Part model, mm, in its own coordinate system. Face numbers are marked on the shaded views. A direction names the side the tool comes from. Round coordinates to 2 decimals unless told otherwise and drop trailing zeros. Loops run counter-clockwise (first coordinate to the right, second up) from the corner with the lowest first, then second, coordinate; pieces in that order, holes last. Notation, with made-up numbers: M -21.5,-2.75 L -3.5,-2.75 A16 cw -3.5,16.25 Z; hole C 21,64 d10. An arc over 180 degrees is marked long. Put each result on its own line as item: value. Start each with the question number.
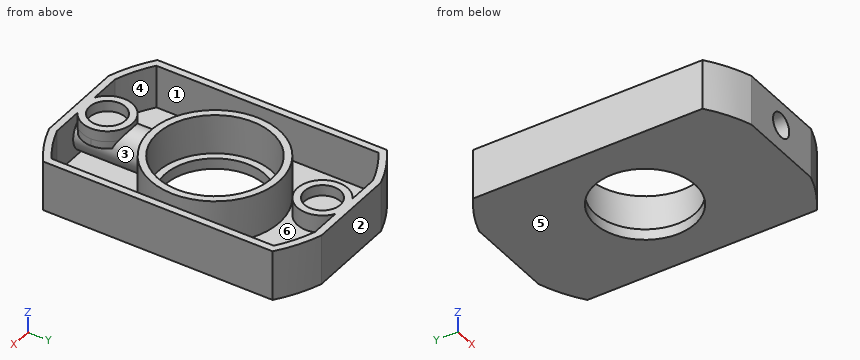
```python
from build123d import *

# Parameters (mm, degrees)
F0_R     = 20
F0_R_2   = 7
F1_DEPTH = 7
F2_R     = 8
F3_DEPTH = 5.5
F4_R     = 2.5
F5_DEPTH = 1.5
F7_DEPTH = 25
F8_R     = 1.7
F9_DEPTH = 10
F10_T    = 1


# Not quite as in the source:
# - a shell that OpenCascade refuses in one call is made with other operations: the cavity is built on its own and cut out


with BuildPart() as f1:
    # F0 (on Top) → F1 (new body)
    with BuildSketch(Plane.XY):
        Circle(F0_R)
        Circle(F0_R_2, mode=Mode.SUBTRACT)
    extrude(amount=F1_DEPTH)

    # F2 (on face) → F3 (cut)
    with BuildSketch(Plane.XY.offset(7)):
        Circle(F2_R)
    extrude(amount=-F3_DEPTH, mode=Mode.SUBTRACT)

    # F4 (on face) → F5 (cut)
    with BuildSketch(Plane.XY.offset(7)):
        with Locations((0, 15)):
            Circle(F4_R)
        with Locations((0, -15)):
            Circle(F4_R)
    extrude(amount=-F5_DEPTH, mode=Mode.SUBTRACT)

    # F6 (on face) → F7 (cut)
    with BuildSketch(Plane.XY.offset(7)):
        with BuildLine():
            Line((-12, -16), (-12, 16))
            ThreePointArc((-12, 16), (-20, 0), (-12, -16))
        make_face()
        with BuildLine():
            Line((12, 16), (12, 19))
            Line((12, 19), (6.2449979984, 19))
            ThreePointArc((6.2449979984, 19), (9.2449979984, 17.7349939952), (12, 16))
        make_face()
        with BuildLine():
            ThreePointArc((-12, 16), (-9.2449979984, 17.7349939952), (-6.2449979984, 19))
            Line((-6.2449979984, 19), (-12, 19))
            Line((-12, 19), (-12, 16))
        make_face()
        with BuildLine():
            Line((12, -19), (12, -16))
            ThreePointArc((12, -16), (9.2449979984, -17.7349939952), (6.2449979984, -19))
            Line((6.2449979984, -19), (12, -19))
        make_face()
        with BuildLine():
            ThreePointArc((-6.2449979984, -19), (-9.2449979984, -17.7349939952), (-12, -16))
            Line((-12, -16), (-12, -19))
            Line((-12, -19), (-6.2449979984, -19))
        make_face()
        with BuildLine():
            ThreePointArc((20, 0), (17.88854382, 8.94427191), (12, 16))
            Line((12, 16), (12, -16))
            ThreePointArc((12, -16), (17.88854382, -8.94427191), (20, 0))
        make_face()
        with BuildLine():
            Line((-6.2449979984, 19), (6.2449979984, 19))
            ThreePointArc((6.2449979984, 19), (0, 20), (-6.2449979984, 19))
        make_face()
        with BuildLine():
            ThreePointArc((-6.2449979984, -19), (0, -20), (6.2449979984, -19))
            Line((6.2449979984, -19), (-6.2449979984, -19))
        make_face()
    extrude(amount=-F7_DEPTH, mode=Mode.SUBTRACT)

    # F8 (on face) → F9 (cut)
    with BuildSketch(Plane.XZ.offset(19)):
        with Locations((0, 3.6865652073)):
            Circle(F8_R)
    extrude(amount=-F9_DEPTH, mode=Mode.SUBTRACT)

    # F10: shell of thickness 1, made by hand


with BuildPart() as f10_core1:
    # F10_t2: copy of F1
    add(f1.part)

    # the walls: a layer under each face that stays
    f10_faces = [f10_core1.faces().sort_by_distance(p)[0] for p in [
        (9.2449979984, 17.7349939952, 3.5),
        (-8, -12.6666666667, 0),
        (0, 19, 3.5),
        (12, 0, 3.5),
        (9.2449979984, -17.7349939952, 3.5),
        (4.1633319989, -19, 1.1666666667),
        (-9.2449979984, -17.7349939952, 3.5),
        (-12, 0, 3.5),
        (-9.2449979984, 17.7349939952, 3.5),
        (-7, 0, 0.75),
        (-2.5, -15, 6.25),
        (-8, 0, 4.25),
        (-2.5, 15, 6.25),
        (-1.7, -14, 3.6865652073),
        (-5.3333333333, -5.3333333333, 1.5),
        (0, -15, 5.5),
        (0, 15, 5.5),
        (0, -9, 3.6865652073),
    ]]
    thicken(f10_faces, amount=-F10_T, mode=Mode.SUBTRACT)

    # F10_s3 → F10_t4 (revolve, cut)
    with BuildSketch(Plane.XZ.offset(15)):
        Polygon((2.49, 5.51), (3.5, 5.5), (3.5, 4.5), (2.5, 4.5), align=None)
    revolve(axis=Axis((0, -15, 5.5), (0, 0, 1)), mode=Mode.SUBTRACT)

    # F10_s5 → F10_t6 (revolve, cut)
    with BuildSketch(Plane.XZ):
        Polygon((7.99, 1.51), (9, 1.5), (9, 0.5), (8, 0.5), align=None)
    revolve(axis=Axis((0, 0, 1.5), (0, 0, 1)), mode=Mode.SUBTRACT)

    # F10_s7 → F10_t8 (revolve, cut)
    with BuildSketch(Plane.XZ.offset(-15)):
        Polygon((2.49, 5.51), (3.5, 5.5), (3.5, 4.5), (2.5, 4.5), align=None)
    revolve(axis=Axis((0, 15, 5.5), (0, 0, 1)), mode=Mode.SUBTRACT)

    # F10_s9 → F10_t10 (revolve, cut)
    with BuildSketch(Plane.XY.offset(3.6865652073)):
        Polygon((1.69, -9.01), (2.7, -9), (2.7, -8), (1.7, -8), align=None)
    revolve(axis=Axis((0, -9, 3.6865652073), (0, -1, 0)), mode=Mode.SUBTRACT)


with BuildPart() as f1_1:
    add(f1.part)

    # what is left inside the walls is the cavity
    f10_cavity = [f10_core1.part.solids().sort_by_distance(p)[0] for p in [
        (5.5, -14, 1.01),
    ]]
    add(f10_cavity, mode=Mode.SUBTRACT)


solid = f1_1.part
```
1. Cut at C-C, the plane z = 3.25. Give the cut face in (x, y) (3 decimals), and give its area (3 significant figures).
2. Cut at B-B, the plane y = 0. Give the cut face in (x, z), and give its area (3 significant figures).
3. Cut at A-A, the plane y = 15. Give the cut face in (x, z), and give its area (3 significant figures).
4. Wall check: L1, parallel to Y at x = 0, z = 1.05; L2, parallel to Y at x = 0, z = 2.5; L3, parallel to Y at x = 0, z = 0.55. Give the ranges that are in metal, low to high.
5. Which spindle directions (+Z, -Z, +X, -X, +Y, -Y) get a long thin tool onto all of the face, cutting with end or side? Do the marked faces 1, 2 and 3. Say none if no direction does.
6. Mould opens along Z. For the marked faces 4, 5 and 6 say: released by +Z, released by -Z, zero draft, split by the parting line, or undercut.
7. Drop flat-ended pins along their axis: pin 1 (1.5 mm diameter, centred on x = 9, y = -14.5, fed in from +Z); pin 2 (4.5 mm diameter, centred on x = 0, y = 15, fed in from +Z); pin 3 (1.7 mm diameter, centred on x = 0, z = 4.5, fed in from -Y). Give the stop position or say it passes through.
8. Cut at D-D, the plane y = -11. Give the cut face in (x, z).
Results list:
1. outline: M -12,-16 A20 ccw -6.245,-19 L -1.643,-19 L -1.643,-9 L 1.643,-9 L 1.643,-19 L 6.245,-19 A20 ccw 12,-16 L 12,16 A20 ccw 6.245,19 L -6.245,19 A20 ccw -12,16 Z; hole M -11,-15.492 A19 ccw -6.083,-18 L -2.664,-18 L -2.664,-8.597 A9 cw long 2.664,-8.597 L 2.664,-18 L 6.083,-18 A19 ccw 11,-15.492 L 11,15.492 A19 ccw 6.083,18 L -6.083,18 A19 ccw -11,15.492 Z; hole C 0,0 d16
1. area: 181 mm^2
2. outline: M -12,0 L -7,0 L -7,1.5 L -8,1.5 L -8,7 L -9,7 L -9,1 L -11,1 L -11,7 L -12,7 Z; M 7,0 L 12,0 L 12,7 L 11,7 L 11,1 L 9,1 L 9,7 L 8,7 L 8,1.5 L 7,1.5 Z
2. area: 35.0 mm^2
3. outline: M -12,0 L 12,0 L 12,7 L 11,7 L 11,1 L -11,1 L -11,7 L -12,7 Z; M -3.5,4.5 L 3.5,4.5 L 3.5,7 L 2.5,7 L 2.5,5.5 L -2.5,5.5 L -2.5,7 L -3.5,7 Z
3. area: 46.0 mm^2
4. L1: y = -19 to -7, 7 to 9, 18 to 19
4. L2: y = -9 to -8, 8 to 9, 18 to 19
4. L3: y = -19 to -7, 7 to 19
5. face 1: +Z
5. face 2: +Z, -Z, +X, -X, +Y
5. face 3: none
6. face 4: zero draft
6. face 5: released by -Z
6. face 6: undercut
7. pin 1: stops at z = 1
7. pin 2: stops at z = 5.5
7. pin 3: stops at y = -9
8. outline: M -12,0 L 12,0 L 12,7 L 11,7 L 11,1 L 0.27,1 A2.7 ccw long -0.27,1 L -11,1 L -11,7 L -12,7 Z; hole C 0,3.69 d3.4
